from build123d import *

# Parameters (mm, degrees)
SKETCH1_R           = 1.75
BOSS_EXTRUDE1_DEPTH = 6
SKETCH2_R           = 2.25
BOSS_EXTRUDE2_DEPTH = 1
CUT_EXTRUDE1_DEPTH  = 1


with BuildPart() as part:
    # Sketch1 → Boss-Extrude1 (new, symmetric)
    with BuildSketch(Plane(origin=(0, 0, 0), x_dir=(1, 0, 0), z_dir=(0, 1, 0))):
        with Locations(Location((0, 0, 0), (0, 0, 270))):
            Circle(SKETCH1_R)
    extrude(amount=BOSS_EXTRUDE1_DEPTH, both=True)

    # Sketch2 → Boss-Extrude2 (add)
    with BuildSketch(Plane(origin=(0, 6, 0), x_dir=(1, 0, 0), z_dir=(0, 1, 0))):
        with Locations(Location((0, 0, 0), (0, 0, 270))):
            Circle(SKETCH2_R)
    extrude(amount=BOSS_EXTRUDE2_DEPTH)

    # Sketch3 → Cut-Extrude1 (cut)
    with BuildSketch(Plane(origin=(0, 7, 0), x_dir=(1, 0, 0), z_dir=(0, 1, 0))):
        Polygon((0.577350272, 1), (1.154700538, -4e-09), (0.577350269, -1.000000006), (-0.577350271, -1.000000002), (-1.15470054, 0), (-0.577350268, 1), align=None)
    extrude(amount=-CUT_EXTRUDE1_DEPTH, mode=Mode.SUBTRACT)


solid = part.part
Source: CAD feature listing. Evaluate the final solid. Frame: model axes, mm. A direction names the side the tool comes from. Coordinates: 2 decimals unless noted, no trailing zeros. Order: outer loops, then holes, each group sorted by start corner. A loop starts at its lowest first (then second) coordinate and runs counter-clockwise, first axis right, second up.
Item 1: Cut plane D-D (x = 0). Return loops of the section in (y, z).
Output values:
outline: (-6, -1.75) - (6, -1.75) - (6, -2.25) - (7, -2.25) - (7, -1) - (6, -1) - (6, 1) - (7, 1) - (7, 2.25) - (6, 2.25) - (6, 1.75) - (-6, 1.75) - close
Item 2: Material intervals for line 1 (Y direction, x = -0.8, z = -1.75); line 2 (X direction, y = 3, z = -0.1); line 3 (Y direction, x = -0.25, z = -0.8), sorted ascending.
Output values:
line 1: y = 6 to 7
line 2: x = -1.75 to 1.75
line 3: y = -6 to 6
Item 3: Cut plane C-C (z = -1.45). Return loops of the section in (x, y).
Output values:
outline: (-1.72, 6) - (-0.98, 6) - (-0.98, -6) - (0.98, -6) - (0.98, 6) - (1.72, 6) - (1.72, 7) - (-1.72, 7) - close
Item 4: Set-up query: faces 1 (the face through (0, -6, 0)), 2 (the face through (-1.71, 0.08, -0.38)), 3 (the face through (0.87, 6.51, 0.49)). Return all of +Z, -Z, +X, -X, +Y, -Y with unobstructed straight access to the full face (end or side cutting, diameter ignored); none if empty.
Output values:
face 1: +Z, -Z, +X, -X, -Y
face 2: -Y
face 3: +Y
Item 5: First-contact query: P1, Ø1.5, axis at y = 4.5, z = 1, coming from the +X side; P2, Ø1.5, axis at x = -1, y = 1.5, coming from the +Z side; P3, Ø1.5, axis at x = 0, y = -1.5, coming from the -Z side. Flat tips, straight axial feed; report the tip coordinate or a pass-through.
Output values:
P1: stops at x = 1.73
P2: stops at z = 1.73
P3: stops at z = -1.75
Item 6: Cut plane A-A (x = 1.45). Return loops of the section in (y, z).
Output values:
outline: (-6, -0.98) - (6, -0.98) - (6, -1.72) - (7, -1.72) - (7, 1.72) - (6, 1.72) - (6, 0.98) - (-6, 0.98) - close
Item 7: Cut plane B-B (y = -2). Return loops of the section in (x, z), plus the area to 3 significant figures.
Output values:
outline: circle Ø3.5 at (0, 0)
area: 9.62 mm2
Item 8: Pull-direction query (Z, two-part tool) for faces 4 (the face through (0, 6.5, 1)), 5 (the face through (-2, 6, 0)), 6 (the face through (0.676, 6.493, 2.146)); classes: pulls with the +Z half, pulls with the -Z half, needs draft (parallel to the pull), parting line crosses it, or undercut.
Output values:
face 4: undercut
face 5: needs draft
face 6: parting line crosses it
